Geometry: final body of the model. Coordinates: model frame, mm. A direction names the side the tool comes from. Coordinates: 2 decimals unless noted, no trailing zeros. Write each loop counter-clockwise with the first axis right and the second up, starting at its lowest first coordinate (ties: lowest second). Pieces come first, ordered by that corner, then holes. Notation, with made-up numbers: (39, 74) - (46, 74) arc R8 cw to (46, 81) - close; hole circle Ø4 at (-38, -6.5). An arc over 180 degrees is marked (long way). Answer as a JSON object with one key per item and string values. Group by question number.
Item 1: Mould query, pull axis Y, two halves, no side actions, for faces 4 (the cylindrical face through (-1.446, -3.525, -0.044)), 5 (the flat face through (-4.5, 0, -6.985)), 6 (the cylindrical face through (-2.74, 2.72, -5.05)). Classes: pulls with the +Y half, pulls with the -Y half, needs draft (parallel to the pull), parting line crosses it, or undercut.
Item 2: Line query: line 1 along Z through (x, y) = (3, 3.25) (3 decimals); line 2 along Z through (x, y) = (0.75, 3.25) (3 decimals); line 3 along Y through (x, z) = (-4.5, -4). Output: solid intervals per line, ascending. Write a range as from..to.
Item 3: Section C-C on y = 1.75. Return loops of the section in (x, z) (3 decimals).
Item 4: Section A-A on x = -1. Return loops of the section in (y, z) (3 decimals), and give its area (3 significant figures).
Item 5: Section B-B on z = -8. Return loops of the section in (x, y).
Item 6: Set-up query: faces 1 (the cylindrical face through (1.47, -3.515, -0.044)), 2 (the cylindrical face through (-3.525, 1.446, -0.044)), 3 (the cylindrical face through (2.74, -2.72, -5.05)). Return all of +Z, -Z, +X, -X, +Y, -Y with unobstructed straight access to the full face (end or side cutting, diameter ignored); none if empty.
Item 7: First-contact query: pin 1 Ø1.3 at (x, y) = (3, -3) entering from -Z (3 decimals); pin 2 Ø1 at (y, z) = (-2.5, 1) entering from +X; pin 3 Ø6 at (x, y) = (1, -2) entering from +Z (3 decimals); pin 4 Ø1.5 at (y, z) = (0.5, 12.5) entering from +X. Flat tips, straight axial feed; report the tip coordinate or a pass-through.
Solid Edge part; units mm, degrees
sketch "Sketch1" plane through (0, 0, 0) normal (0, 0, 1) x (1, 0, 0)
  arc A0 (-0.5843, 4.4447) -> (0, 5.0777) centre (0.0507, 4.4447) cw
  arc A1 (0.5843, 4.4447) -> (0, 5.0777) centre (-0.0507, 4.4447) ccw
  line L0 (0.5843, 3.7649) -> (0.5843, 4.4447)
  arc A2 (2.249, 3.0754) -> (0.5843, 3.7649) centre (0, 0) ccw
  line L1 (2.249, 3.0754) -> (2.7297, 3.5561)
  arc A3 (2.7297, 3.5561) -> (3.5905, 3.5905) centre (3.1787, 3.1071) cw
  arc A4 (3.5561, 2.7297) -> (3.5905, 3.5905) centre (3.1071, 3.1787) ccw
  line L2 (3.0754, 2.249) -> (3.5561, 2.7297)
  arc A5 (3.7649, 0.5843) -> (3.0754, 2.249) centre (0, 0) ccw
  line L3 (3.7649, 0.5843) -> (4.4447, 0.5843)
  arc A6 (4.4447, 0.5843) -> (5.0777, 0) centre (4.4447, -0.0507) cw
  arc A7 (4.4447, -0.5843) -> (5.0777, 0) centre (4.4447, 0.0507) ccw
  line L4 (3.7689, -0.5843) -> (4.4447, -0.5843)
  line L5 (3.7625, -0.5998) -> (3.7689, -0.5843)
  arc A8 (3.7625, -0.5998) -> (3.0754, -2.249) centre (0, 0) cw
  line L6 (3.0754, -2.249) -> (3.5561, -2.7297)
  arc A9 (3.5561, -2.7297) -> (3.5905, -3.5905) centre (3.1071, -3.1787) cw
  arc A10 (2.7297, -3.5561) -> (3.5905, -3.5905) centre (3.1787, -3.1071) ccw
  line L7 (2.249, -3.0754) -> (2.7297, -3.5561)
  arc A11 (2.249, -3.0754) -> (0.5843, -3.7649) centre (0, 0) cw
  line L8 (0.5843, -3.7649) -> (0.5843, -4.4447)
  arc A12 (0.5843, -4.4447) -> (0, -5.0777) centre (-0.0507, -4.4447) cw
  arc A13 (-0.5843, -4.4447) -> (0, -5.0777) centre (0.0507, -4.4447) ccw
  line L9 (-0.5843, -3.7649) -> (-0.5843, -4.4447)
  arc A14 (-0.5843, -3.7649) -> (-2.249, -3.0754) centre (0, 0) cw
  line L10 (-2.249, -3.0754) -> (-2.7297, -3.5561)
  arc A15 (-2.7297, -3.5561) -> (-3.5905, -3.5905) centre (-3.1787, -3.1071) cw
  arc A16 (-3.5561, -2.7297) -> (-3.5905, -3.5905) centre (-3.1071, -3.1787) ccw
  line L11 (-3.0754, -2.249) -> (-3.5561, -2.7297)
  arc A17 (-3.0754, -2.249) -> (-3.7649, -0.5843) centre (0, 0) cw
  line L12 (-3.7649, -0.5843) -> (-4.4447, -0.5843)
  arc A18 (-4.4447, -0.5843) -> (-5.0777, 0) centre (-4.4447, 0.0507) cw
  arc A19 (-4.4447, 0.5843) -> (-5.0777, 0) centre (-4.4447, -0.0507) ccw
  line L13 (-3.7649, 0.5843) -> (-4.4447, 0.5843)
  arc A20 (-3.7649, 0.5843) -> (-3.0754, 2.249) centre (0, 0) cw
  line L14 (-3.0754, 2.249) -> (-3.5561, 2.7297)
  arc A21 (-3.5561, 2.7297) -> (-3.5905, 3.5905) centre (-3.1071, 3.1787) cw
  arc A22 (-2.7297, 3.5561) -> (-3.5905, 3.5905) centre (-3.1787, 3.1071) ccw
  line L15 (-2.249, 3.0754) -> (-2.7297, 3.5561)
  arc A23 (-2.249, 3.0754) -> (-0.5843, 3.7649) centre (0, 0) cw
  line L16 (-0.5843, 3.7649) -> (-0.5843, 4.4447)
extrude "Protrusion1" add sketch "Sketch1" along normal mid plane 6.35
sketch "Sketch2" plane through (0, 0, 0) normal (0, 0, 1) x (1, 0, 0)
  arc A0 (3.5561, 2.7297) -> (3.5905, 3.5905) centre (3.1071, 3.1787) ccw
  arc A1 (2.7297, 3.5561) -> (3.5905, 3.5905) centre (3.1787, 3.1071) cw
  arc A2 (3.5561, 2.7297) -> (2.7297, 3.5561) centre (3.1429, 3.1429) cw
  arc A3 (4.4447, 0.5843) -> (4.4447, -0.5843) centre (4.4447, 0) ccw
  arc A4 (4.4447, -0.5843) -> (5.0777, 0) centre (4.4447, 0.0507) ccw
  arc A5 (4.4447, 0.5843) -> (5.0777, 0) centre (4.4447, -0.0507) cw
  arc A6 (3.5561, -2.7297) -> (2.7297, -3.5561) centre (3.1429, -3.1429) ccw
  arc A7 (2.7297, -3.5561) -> (3.5905, -3.5905) centre (3.1787, -3.1071) ccw
  arc A8 (3.5561, -2.7297) -> (3.5905, -3.5905) centre (3.1071, -3.1787) cw
  arc A9 (0.5843, -4.4447) -> (0, -5.0777) centre (-0.0507, -4.4447) cw
  arc A10 (-0.5843, -4.4447) -> (0, -5.0777) centre (0.0507, -4.4447) ccw
  arc A11 (0.5843, -4.4447) -> (-0.5843, -4.4447) centre (0, -4.4447) ccw
  arc A12 (-2.7297, -3.5561) -> (-3.5561, -2.7297) centre (-3.1429, -3.1429) ccw
  arc A13 (-3.5561, -2.7297) -> (-3.5905, -3.5905) centre (-3.1071, -3.1787) ccw
  arc A14 (-2.7297, -3.5561) -> (-3.5905, -3.5905) centre (-3.1787, -3.1071) cw
  arc A15 (-4.4447, 0.5843) -> (-4.4447, -0.5843) centre (-4.4447, 0) cw
  arc A16 (-4.4447, -0.5843) -> (-5.0777, 0) centre (-4.4447, 0.0507) cw
  arc A17 (-4.4447, 0.5843) -> (-5.0777, 0) centre (-4.4447, -0.0507) ccw
  arc A18 (-2.7297, 3.5561) -> (-3.5905, 3.5905) centre (-3.1787, 3.1071) ccw
  arc A19 (-3.5561, 2.7297) -> (-3.5905, 3.5905) centre (-3.1071, 3.1787) cw
  arc A20 (-2.7297, 3.5561) -> (-3.5561, 2.7297) centre (-3.1429, 3.1429) cw
  arc A21 (0.5843, 4.4447) -> (-0.5843, 4.4447) centre (0, 4.4447) cw
  arc A22 (-0.5843, 4.4447) -> (0, 5.0777) centre (0.0507, 4.4447) cw
  arc A23 (0.5843, 4.4447) -> (0, 5.0777) centre (-0.0507, 4.4447) ccw
extrude "ExtrudedProtrusion_2" add sketch "Sketch2" against normal blind 6.985
sketch "Sketch3" plane through (0, 0, -3.175) normal (0, 0, -1) x (0, 1, 0)
  circle A0 centre (0, 0) radius 1.27
extrude "ExtrudedProtrusion_3" add sketch "Sketch3" along normal blind 8.89
sketch "Sketch4" plane through (0, 0, 3.175) normal (0, 0, 1) x (0, 1, 0)
  circle A0 centre (0, 0) radius 1.27
extrude "ExtrudedProtrusion_4" add sketch "Sketch4" along normal blind 15.24
Checks:
{
 "1": {"face 4": "pulls with the -Y half", "face 5": "needs draft", "face 6": "undercut"},
 "2": {"line 1": "-6.985..3.175", "line 2": "-3.175..3.175", "line 3": "-0.58..0.58"},
 "3": {"outline": "(-3.384, -3.175) - (3.384, -3.175) - (3.384, 3.175) - (-3.384, 3.175) - close"},
 "4": {"outline": "(-3.676, -3.175) - (-0.783, -3.175) - (-0.783, -12.065) - (0.783, -12.065) - (0.783, -3.175) - (3.676, -3.175) - (3.676, 3.175) - (0.783, 3.175) - (0.783, 18.415) - (-0.783, 18.415) - (-0.783, 3.175) - (-3.676, 3.175) - close", "area": "84.5 mm^2"},
 "5": {"outline": "circle Ø2.54 at (0, 0)"},
 "6": {"face 1": "+Z, -Z, -Y", "face 2": "+Z, -Z, -X", "face 3": "-Z"},
 "7": {"pin 1": "z = -6.985", "pin 2": "x = 3.72", "pin 3": "z = 18.415", "pin 4": "x = 1.27"}
}
